```python
from build123d import *

# Parameters (mm, degrees)
F0_W     = 736.6
F0_H     = 562.991
F0_W_2   = 711.2
F0_H_2   = 537.591
F1_DEPTH = 812.8
F2_DEPTH = 787.4


with BuildPart() as f1:
    # F0 (on Front) → F1 (new body)
    with BuildSketch(Plane.XZ):
        Rectangle(F0_W, F0_H)
        Rectangle(F0_W_2, F0_H_2, mode=Mode.SUBTRACT)
        Rectangle(F0_W_2, F0_H_2)
    extrude(amount=-F1_DEPTH)

    # F0 (on Front) → F2 (cut)
    with BuildSketch(Plane.XZ):
        Rectangle(F0_W_2, F0_H_2)
    extrude(amount=-F2_DEPTH, mode=Mode.SUBTRACT)


solid = f1.part
```
For this review, take the finished solid that the model builds, in its own axes (mm). A direction names the side the tool comes from. Round coordinates to 2 decimals unless told otherwise and drop trailing zeros. Write each loop counter-clockwise with the first axis right and the second up, starting at its lowest first coordinate (ties: lowest second). Pieces come first, ordered by that corner, then holes. Notation, with made-up numbers: (-7, -25.5) -> (19, -25.5) arc R4 cw to (19, -18.5) -> close; hole circle Ø5 at (-7, 17.5). An arc over 180 degrees is marked (long way). Use one line per item in the form item = value.
1) Take a section at C-C, the plane z = -161.5. Write out the cut boundary in (x, y).
Found:
outline = (-368.3, 0) -> (-355.6, 0) -> (-355.6, 787.4) -> (355.6, 787.4) -> (355.6, 0) -> (368.3, 0) -> (368.3, 812.8) -> (-368.3, 812.8) -> close
2) Take a section at A-A, the plane y = 614.5. Write out the cut boundary in (x, z), and give its area (3 significant figures).
Found:
outline = (-368.3, -281.5) -> (368.3, -281.5) -> (368.3, 281.5) -> (-368.3, 281.5) -> close; hole (-355.6, -268.8) -> (355.6, -268.8) -> (355.6, 268.8) -> (-355.6, 268.8) -> close
area = 32,400 mm2
3) Take a section at B-B, the plane x = -225. Write out the cut boundary in (y, z), and give its area (3 significant figures).
Found:
outline = (0, -281.5) -> (812.8, -281.5) -> (812.8, 281.5) -> (0, 281.5) -> (0, 268.8) -> (787.4, 268.8) -> (787.4, -268.8) -> (0, -268.8) -> close
area = 34,300 mm2
4) To check wall thickness, follow L1, parallel to Z at x = 172, y = 777; L2, parallel to X at y = 284.5, z = -27.5; L3, parallel to Y at x = -230.5, z = -245. State the ranges of each line that lie inside material, in increasing order. Write a range as from..to.
Found:
L1 = -281.5..-268.8, 268.8..281.5
L2 = -368.3..-355.6, 355.6..368.3
L3 = 787.4..812.8
5) Tool access review of faces 4 (the flat face through (-356, 0, 1)), 5 (the flat face through (-5, 388, -268.796)): name each direction out of +Z, -Z, +X, -X, +Y, -Y from which nothing blocks a thin tool from reaching the whole face with its end or side.
Found:
face_4 = +Z, -Z, +X, -X, -Y
face_5 = -Y
6) Mouldability with a two-part tool opening along Z and no side actions: class faces 1 (the flat face through (-355.6, 388, -4)), 2 (the flat face through (-5, 812.8, 4)), 3 (the flat face through (-5, 401, -281.496)) as +Z half, -Z half, draft (parallel to the pull), parting line (faces both ways), or undercut.
Found:
face_1 = undercut
face_2 = draft
face_3 = -Z half
